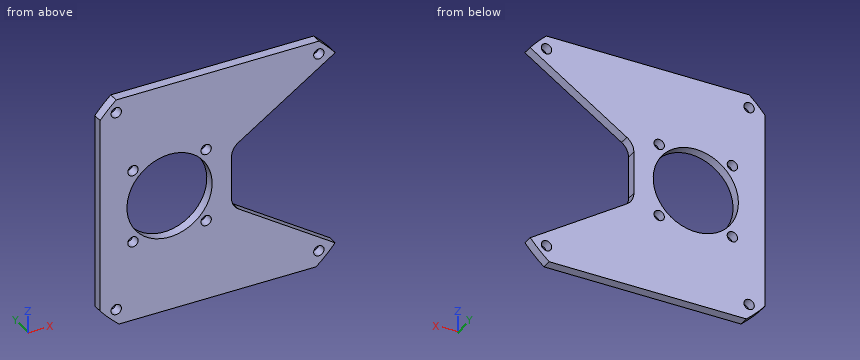
```python
from build123d import *

# Parameters (mm, degrees)
SKETCH1_R            = 13.97
BOSS_EXTRUDE1_DEPTH  = 1.5875
FILLET1_R            = 5.08
M3_CLEARANCE_HOLE1_D = 3.4
M3_CLEARANCE_HOLE2_D = 3.4


with BuildPart() as part:
    # Sketch1 → Boss-Extrude1 (new, symmetric)
    with BuildSketch(Plane(origin=(0, 0, 0), x_dir=(1, 0, 0), z_dir=(0, 1, 0))):
        with BuildLine():
            Line((-38.50947489, 32.14883464), (-38.50947489, -32.14883464))
            ThreePointArc((-38.50947489, -32.14883464), (-35.992876625, -34.943383598), (-33.274, -37.541552299))
            Line((-33.274, -37.541552299), (33.274, -37.541552299))
            ThreePointArc((33.274, -37.541552299), (36.035191498, -34.899744966), (38.587271968, -32.055415565))
            Line((38.587271968, -32.055415565), (4.572, -9.720985565))
            Line((4.572, -9.720985565), (4.572, 9.720985565))
            Line((4.572, 9.720985565), (38.541369471, 32.110591154))
            ThreePointArc((38.541369471, 32.110591154), (35.567819018, 35.375944868), (32.318597457, 38.367114609))
            Line((32.318597457, 38.367114609), (-32.318597457, 38.367114609))
            ThreePointArc((-32.318597457, 38.367114609), (-35.55025611, 35.393594272), (-38.50947489, 32.14883464))
        make_face()
        with Locations(Location((-15.748, 0, 0), (0, 0, 270))):
            Circle(SKETCH1_R, mode=Mode.SUBTRACT)
    extrude(amount=BOSS_EXTRUDE1_DEPTH, both=True)

    # Fillet1
    fillet1_edges = [part.edges().sort_by_distance(p)[0] for p in [
        (4.572, 0, -9.720985565),
        (4.572, 0, 9.720985565),
    ]]
    fillet(fillet1_edges, radius=FILLET1_R)

    # M3 Clearance Hole1 (through all)
    with Locations(Plane(origin=(0, 1.5875, 0), x_dir=(1, 0, 0), z_dir=(0, 1, 0))):
        with Locations((-33.226947648, 33.226947648), (33.226947648, 33.226947648), (33.226947648, -33.226947648), (-33.226947648, -33.226947648)):
            Hole(M3_CLEARANCE_HOLE1_D / 2)

    # M3 Clearance Hole2 (through all)
    with Locations(Plane(origin=(0, 1.5875, 0), x_dir=(1, 0, 0), z_dir=(0, 1, 0))):
        with Locations((-27.748, 12), (-3.748, 12), (-3.748, -12), (-27.748, -12)):
            Hole(M3_CLEARANCE_HOLE2_D / 2)


solid = part.part
```
Check sheet for the modelled part. Datum: model origin and axes. Units: mm. Coordinates: 2 decimals unless noted, no trailing zeros. Loops run counter-clockwise (first coordinate to the right, second up) from the corner with the lowest first, then second, coordinate; pieces in that order, holes last. Notation, with made-up numbers: M -38.5,-5 L 11.5,-5 A18 cw 11.5,4 Z; hole C -11.75,82.25 d1. An arc over 180 degrees is marked long. Answer as a JSON object with one key per item and string values.
1. Sectioned sample at A-A on z = 0. Record the cut outline in (x, y), and give its area (3 significant figures).
Outcome:
{"outline": "M -38.51,-1.59 L -29.72,-1.59 L -29.72,1.59 L -38.51,1.59 Z; M -1.78,-1.59 L 4.57,-1.59 L 4.57,1.59 L -1.78,1.59 Z", "area": "48.1 mm²"}
2. Sectioned sample at B-B on x = -21. Record the cut outline in (y, z).
Outcome:
{"outline": "M -1.59,-38.37 L 1.59,-38.37 L 1.59,-12.95 L -1.59,-12.95 Z; M -1.59,12.95 L 1.59,12.95 L 1.59,37.54 L -1.59,37.54 Z"}
3. Depth check by flat-ended pin: P1, Ø2, axis at x = -3.748, z = -12, coming from the +Y side; P2, Ø1.6, axis at y = 0, z = -1, coming from the +X side; P3, Ø1, axis at y = 1, z = -12, coming from the +X side. Enter the tip coordinate at first touch or a pass-through.
Outcome:
{"P1": "through", "P2": "x = 4.57", "P3": "x = 8.79"}
4. Sectioned sample at C-C on y = 0.9. Count the separate pieces of the cut face and the enclosed holes in it, and give its area (3 significant figures).
Outcome:
{"separate pieces": "1", "enclosed holes": "9", "area": "3,680 mm²"}
5. Scan lines: L1, parallel to X at y = -0.4, z = 0; L2, parallel to X at y = 0.6, z = 11; L3, parallel to X at y = -0.5, z = 10.5. Record each from-to range of solid material in increasing order. Write a range as from..to.
Outcome:
{"L1": "-38.51..-29.72, -1.78..4.57", "L2": "-38.51..-29.12, -26.37..-24.36, -7.14..-5.12, -2.37..6.55", "L3": "-38.51..-28.55, -26.95..-24.96, -6.53..-4.55, -2.95..5.99"}
